Build history of the part. All positions in model axes, mm. Face numbers are marked on the shaded views. A direction names the side the tool comes from. Give positions to 0.01 mm unless a question says otherwise; leave off trailing zeros. Write each loop counter-clockwise with the first axis right and the second up, starting at its lowest first coordinate (ties: lowest second). Pieces come first, ordered by that corner, then holes.
from build123d import *

# Parameters (mm, degrees)
SKETCH1_R           = 1.5
BOSS_EXTRUDE1_DEPTH = 1.4
SKETCH2_R           = 1.15
BOSS_EXTRUDE2_DEPTH = 0.6
SKETCH3_R           = 1.5
BOSS_EXTRUDE3_DEPTH = 4
REVOLVE1_ANGLE      = 180
CHAMFER1_SIZE       = 0.25


with BuildPart() as part:
    # Sketch1 → Boss-Extrude1 (new body)
    with BuildSketch(Plane.XY):
        Circle(SKETCH1_R)
    extrude(amount=BOSS_EXTRUDE1_DEPTH)

    # Sketch2 → Boss-Extrude2 (add)
    with BuildSketch(Plane.XY.offset(1.4)):
        Circle(SKETCH2_R)
    extrude(amount=BOSS_EXTRUDE2_DEPTH)

    # Sketch3 → Boss-Extrude3 (add)
    with BuildSketch(Plane.XY.offset(2)):
        Circle(SKETCH3_R)
    extrude(amount=BOSS_EXTRUDE3_DEPTH)

    # Sketch4 → Revolve1 (revolve)
    with BuildSketch(Plane.XY.offset(6)):
        with BuildLine():
            Line((0, 2), (0, -2))
            ThreePointArc((0, -2), (2, 0), (0, 2))
        make_face()
    revolve(axis=Axis((0, 2, 6), (0, -1, 0)), revolution_arc=REVOLVE1_ANGLE)

    # Chamfer1
    chamfer1_edges = [part.edges().sort_by_distance(p)[0] for p in [
        (-1.5, 0, 0),
    ]]
    chamfer(chamfer1_edges, length=CHAMFER1_SIZE)


solid = part.part
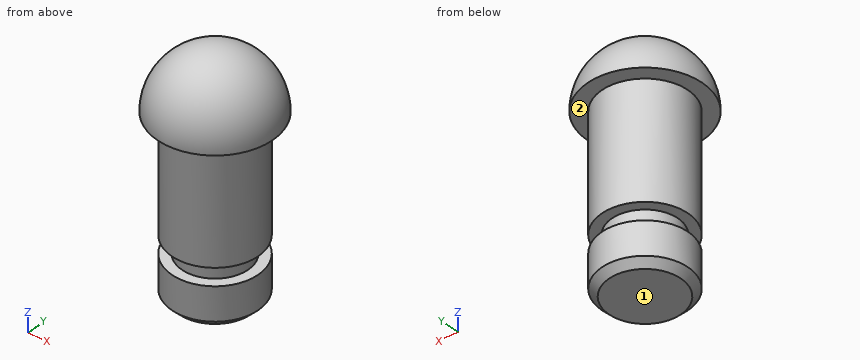
(1) Saw through at D-D, the plane y = 1.6. List the corners of the cut face in (x, z), plus the area to 3 significant figures.
(2) Saw through at C-C, the plane z = 2.5. List the corners of the cut face in (x, y), plus the area to 3 significant figures.
(3) 3-axis set-ups, long thin cutter, end or side, ignore diameter. For the marked faces 1 and 2: which of +Z, -Z, +X, -X, +Y, -Y reach the whole face in a straight line?
(4) Probe line 1 (X direction, y = -0.5, z = 3); line 2 (Z direction, x = 0.8, y = 0.45); line 3 (Y direction, x = 0.8, z = 1.75). List the from-to ranges inside material, lowest first.
(5) Saw through at A-A, the plane x = 0. List the corners of the cut face in (y, z).
(6) Drop a flat-ended pin along its axis: pin 1 (1.5 mm diameter, centred on x = 0.5, z = 3.5, fed in from +Y). Give the stop position or say it passes through.
Computed values:
1. outline: (-1.2, 6) - (1.2, 6) arc R1.2 ccw to start
1. area: 2.26 mm2
2. outline: circle Ø3 at (0, 0)
2. area: 7.07 mm2
3. face 1: -Z, +X, -X, +Y, -Y
3. face 2: -Z
4. line 1: x = -1.41 to 1.41
4. line 2: z = 0 to 7.78
4. line 3: y = -0.83 to 0.83
5. outline: (-2, 6) - (-1.5, 6) - (-1.5, 2) - (-1.15, 2) - (-1.15, 1.4) - (-1.5, 1.4) - (-1.5, 0.25) - (-1.25, 0) - (1.25, 0) - (1.5, 0.25) - (1.5, 1.4) - (1.15, 1.4) - (1.15, 2) - (1.5, 2) - (1.5, 6) - (2, 6) arc R2 ccw to start
6. pin 1: stops at y = 1.5
